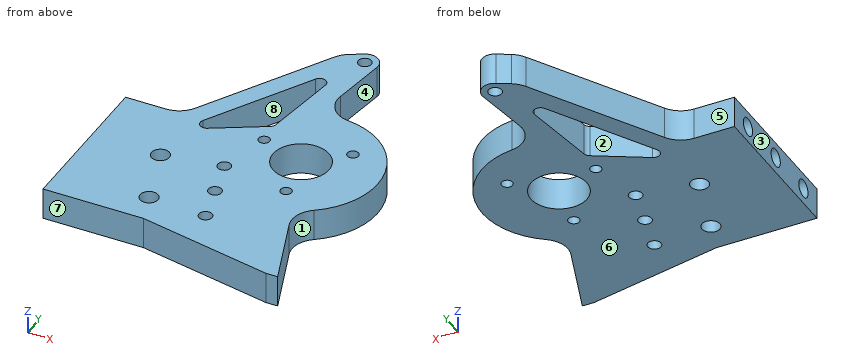
```python
from build123d import *

# Parameters (mm, degrees)
ESBO_O1_R                                   = 10.6
RESSALTO_EXTRUS_O1_DEPTH                    = 12
FILETE1_R                                   = 10
CORTE_EXTRUS_O1_DEPTH                       = 161.30276936
FILETE3_R                                   = 2.5
CORTE_EXTRUS_O2_DEPTH                       = 161.30276936
BROCA_DE_ROSQUEAR_PARA_TARRAXA_DE_M81_D     = 6.8
BROCA_DE_ROSQUEAR_PARA_TARRAXA_DE_M81_DEPTH = 15
BROCA_DE_ROSQUEAR_PARA_TARRAXA_DE_M81_TIP   = 2.042926105
FILETE6_R                                   = 10
FILETE7_R                                   = 5
BROCA_DE_ROSQUEAR_PARA_TARRAXA_DE_M61_D     = 5
BROCA_DE_ROSQUEAR_PARA_TARRAXA_DE_M82_D     = 6.8
BROCA_DE_ROSQUEAR_PARA_TARRAXA_DE_M51_D     = 4.2
BROCA_DE_ROSQUEAR_PARA_TARRAXA_DE_M62_D     = 5


with BuildPart() as part:
    # Esboço1 → Ressalto-extrusão1 (new body)
    with BuildSketch(Plane.XY):
        with BuildLine():
            Line((0, 0), (36, 0))
            Line((36, 0), (36, -10))
            Line((36, -10), (94, -10))
            Line((94, -10), (80.53931892, 26.982917317))
            ThreePointArc((80.53931892, 26.982917317), (97.53650317, 63.096207626), (62.372346743, 81.978901083))
            Line((62.372346743, 81.978901083), (68.8, 125.506883733))
            Line((68.8, 125.506883733), (53, 116.345625842))
            Line((53, 116.345625842), (21, 60.92))
            Line((21, 60.92), (0, 60.92))
            Line((0, 60.92), (0, 0))
        make_face()
        with Locations((70, 54)):
            Circle(ESBO_O1_R, mode=Mode.SUBTRACT)
    extrude(amount=RESSALTO_EXTRUS_O1_DEPTH)

    # Filete1
    filete1_edges = [part.edges().sort_by_distance(p)[0] for p in [
        (21, 60.92, 6),
        (53, 116.345625842, 6),
        (62.372346743, 81.978901083, 6),
    ]]
    fillet(filete1_edges, radius=FILETE1_R)

    # Esboço2 → Corte-extrusão1 (cut, through all)
    with BuildSketch(Plane.XY.offset(12)):
        Polygon((24.783390445, 52.473024476), (58.570061959, 110.993256157), (52.283390445, 68.42), align=None)
    extrude(amount=-CORTE_EXTRUS_O1_DEPTH, mode=Mode.SUBTRACT)

    # Filete3
    filete3_edges = [part.edges().sort_by_distance(p)[0] for p in [
        (52.283390445, 68.42, 6),
        (24.783390445, 52.473024476, 6),
        (58.570061959, 110.993256157, 6),
    ]]
    fillet(filete3_edges, radius=FILETE3_R)

    # Esboço8 → Corte-extrusão2 (cut, through all)
    with BuildSketch(Plane.XY.offset(12)):
        Polygon((89.5, -10), (38, 0), (36, 0), (36, -10), align=None)
    extrude(amount=-CORTE_EXTRUS_O2_DEPTH, mode=Mode.SUBTRACT)

    # Broca de rosquear para tarraxa de M81
    with Locations(Plane.ZY):
        with Locations((6, 50.92), (6, 30.46), (6, 10)):
            Hole(BROCA_DE_ROSQUEAR_PARA_TARRAXA_DE_M81_D / 2, depth=BROCA_DE_ROSQUEAR_PARA_TARRAXA_DE_M81_DEPTH)
            with Locations((0, 0, -(BROCA_DE_ROSQUEAR_PARA_TARRAXA_DE_M81_DEPTH + BROCA_DE_ROSQUEAR_PARA_TARRAXA_DE_M81_TIP / 2))):  # 118° drill point
                Cone(0, BROCA_DE_ROSQUEAR_PARA_TARRAXA_DE_M81_D / 2, BROCA_DE_ROSQUEAR_PARA_TARRAXA_DE_M81_TIP, mode=Mode.SUBTRACT)

    # Filete6
    filete6_edges = [part.edges().sort_by_distance(p)[0] for p in [
        (80.53931892, 26.982917317, 6),
    ]]
    fillet(filete6_edges, radius=FILETE6_R)

    # Filete7
    filete7_edges = [part.edges().sort_by_distance(p)[0] for p in [
        (68.8, 125.506883733, 6),
    ]]
    fillet(filete7_edges, radius=FILETE7_R)

    # Broca de rosquear para tarraxa de M61 (through all)
    with Locations(Plane.XY.offset(12)):
        with Locations((48.161384096, 39.952181527), (52.043669773, 25.463294133), (55.925955449, 10.974406739)):
            Hole(BROCA_DE_ROSQUEAR_PARA_TARRAXA_DE_M61_D / 2)

    # Broca de rosquear para tarraxa de M82 (through all)
    with Locations(Plane.XY.offset(12)):
        with Locations((26, 35.952181527), (34, 12)):
            Hole(BROCA_DE_ROSQUEAR_PARA_TARRAXA_DE_M82_D / 2)

    # Broca de rosquear para tarraxa de M51 (through all)
    with Locations(Plane.XY.offset(12)):
        with Locations((83.600921147, 65.790459871), (73.410377197, 36.326026837), (52.988701656, 59.883513293)):
            Hole(BROCA_DE_ROSQUEAR_PARA_TARRAXA_DE_M51_D / 2)

    # Broca de rosquear para tarraxa de M62 (through all)
    with Locations(Plane.XY.offset(12)):
        with Locations((62.339118507, 115.980990674)):
            Hole(BROCA_DE_ROSQUEAR_PARA_TARRAXA_DE_M62_D / 2)


solid = part.part
```
Could you check a few things on this model? Use its own coordinates, in mm. Face numbers are marked on the shaded views. A direction names the side the tool comes from. Round coordinates to 2 decimals unless told otherwise and drop trailing zeros. Loops run counter-clockwise (first coordinate to the right, second up) from the corner with the lowest first, then second, coordinate; pieces in that order, holes last. Notation, with made-up numbers: (74.25, 41) - (89.25, 41) arc R12 cw to (89.25, 50) - close; hole circle Ø6 at (-18.5, -28.75). An arc over 180 degrees is marked (long way). Answer in a Markdown table with one row per item. Add a question column.
(1) If we section it at B-B (x = 26): Please give me the cut outline in (y, z), plus the area to 3 significant figures.
(2) I need wall thicknesses on line 1 along Y through (x, z) = (11, 6); line 2 along Z through (x, y) = (4, 30.46); line 3 along Y through (x, z) = (12.5, 6.5). Which ranges of each line are inside material? Lowest first, please.
(3) If we mould it in two halves opening along X, with no side actions, what happens to the marked faces 1, 2 and 3? For each: pulls with the +X half, pulls with the -X half, needs draft (parallel to the pull), parting line crosses it, or undercut.
(4) If we section it at C-C (z = 7.75): State how many separate pieces and enclosed holes the cut face has, plus the area to 3 significant figures.
(5) If we section it at A-A (y = 73.5): Please give me the cut outline in (x, z).
(6) I'm going to push flat-ended pins straight in: pin 1 (4.5 mm diameter, centred on x = 55.93, y = 10.97, fed in from +Z); pin 2 (3.5 mm diameter, centred on x = 4, z = 6, fed in from +Y); pin 3 (2 mm diameter, centred on y = 10, z = 5, fed in from -X); pin 4 (1.5 mm diameter, centred on y = 39.5, z = 7, fed in from +X). Where does each tip first touch, or does it pass through?
(7) For the marked faces 4, 5, 6, 7 and 8, which set-ups out of +Z, -Z, +X, -X, +Y, -Y let a thin tool reach every point of the face, with its end or its side?
Model answer:
| question | item | result |
|---|---|---|
| 1 | outline | (0, 0) - (32.55, 0) - (32.55, 12) - (0, 12) - close; (39.35, 0) - (69.58, 0) - (69.58, 12) - (39.35, 12) - close |
| 1 | area | 753 mm² |
| 2 | line 1 | y = 0 to 6.6, 13.4 to 27.06, 33.86 to 47.52, 54.32 to 60.92 |
| 2 | line 2 | z = 0 to 2.6, 9.4 to 12 |
| 2 | line 3 | y = 0 to 6.64, 13.36 to 27.1, 33.82 to 47.56, 54.28 to 60.92 |
| 3 | face 1 | pulls with the +X half |
| 3 | face 2 | undercut |
| 3 | face 3 | pulls with the -X half |
| 4 | separate pieces | 1 |
| 4 | enclosed holes | 11 |
| 4 | area | 6,710 mm² |
| 5 | outline | (28.26, 0) - (36.92, 0) - (36.92, 12) - (28.26, 12) - close; (53.03, 0) - (91.47, 0) - (91.47, 12) - (53.03, 12) - close |
| 6 | pin 1 | passes through |
| 6 | pin 2 | stops at y = 60.92 |
| 6 | pin 3 | stops at x = 15.84 |
| 6 | pin 4 | stops at x = 95.53 |
| 7 | face 4 | +Z, -Z, +X |
| 7 | face 5 | +Z, -Z, -X, +Y |
| 7 | face 6 | -Z, +X, -X, +Y, -Y |
| 7 | face 7 | +Z, -Z, -X, -Y |
| 7 | face 8 | +Z, -Z |
